Geometry: see drawing. Coordinates: mm, zero at the bounding-box minimum. A direction names the side the tool comes from. Round coordinates to 2 decimals unless told otherwise and drop trailing zeros. Order: outer loops, then holes, each group sorted by start corner. A loop starts at its lowest first (then second) coordinate and runs counter-clockwise, first axis right, second up. Notation, with made-up numbers: (-34, 24) -> (7, 24) arc R21 cw to (7, 36) -> close; hole circle Ø5 at (-32.75, 74). An arc over 180 degrees is marked (long way). Use a Markdown table: item, result.
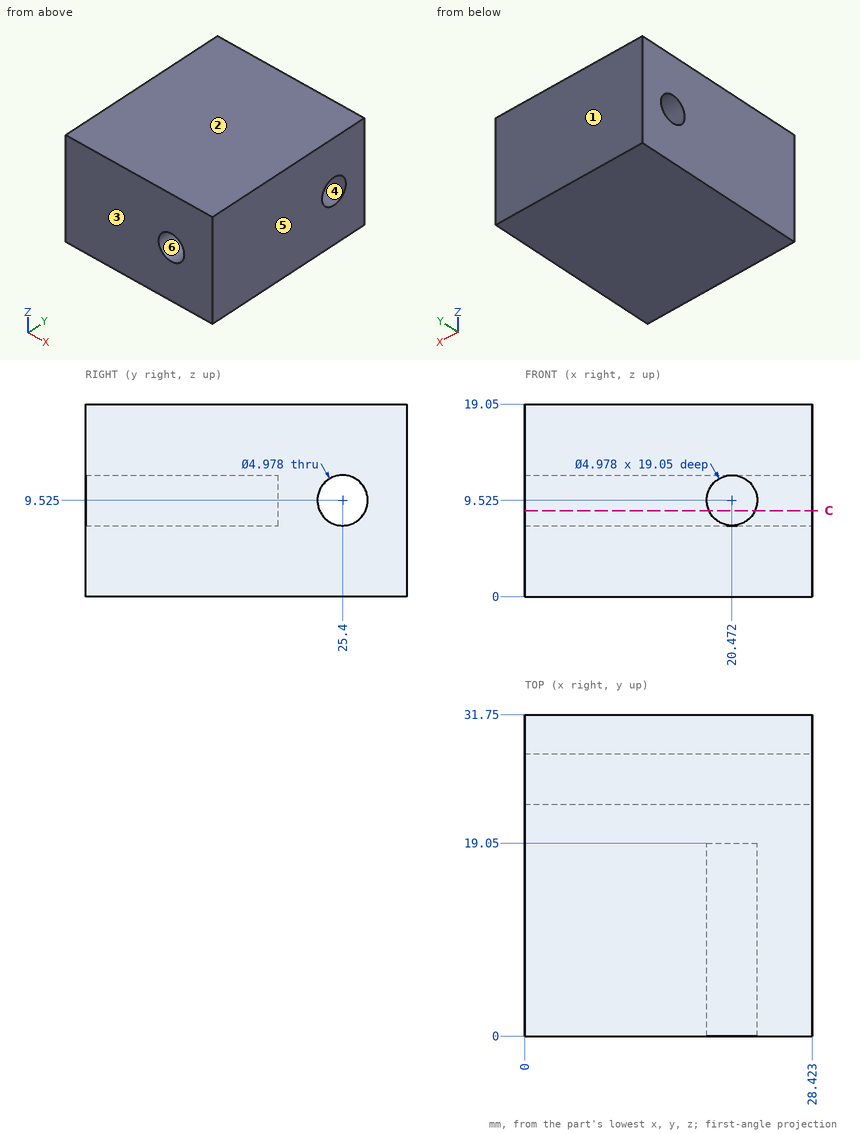
1) Contact query for a flat-ended pin moving along its axis: P1, Ø2.5, axis at x = 19.5, z = 9, coming from the -Y side. Output: stop coordinate, or through.
Answer key:
| item | result |
|---|---|
| P1 | stops at y = 19.05 |
2) Draft query along Y for the marked faces 1, 2, 3 and 4. Return one class per face: released by +Y, released by -Y, zero draft, split by the parting line, or undercut.
Answer key:
| item | result |
|---|---|
| face 1 | released by +Y |
| face 2 | zero draft |
| face 3 | released by -Y |
| face 4 | undercut |
3) Set-up query: the marked faces 5 and 6. Return all of +Z, -Z, +X, -X, +Y, -Y with unobstructed straight access to the full face (end or side cutting, diameter ignored); none if empty.
Answer key:
| item | result |
|---|---|
| face 5 | +Z, -Z, +X, +Y, -Y |
| face 6 | -Y |
4) Ray query, probe 1 along Z at (x, y) = (18.75, 25.5); probe 2 along Y at (x, z) = (12.5, 9); probe 3 along X at (y, z) = (3.5, 9) (1 decimal). Return the intervals inside material, ascending.
Answer key:
| item | result |
|---|---|
| probe 1 | z = 0 to 7.04, 12.01 to 19.05 |
| probe 2 | y = 0 to 22.97, 27.83 to 31.75 |
| probe 3 | x = 0 to 18, 22.9 to 28.4 |
5) Cut plane C-C on z = 8.5. Return loops of the section in (x, y), and give its area (3 significant figures).
Answer key:
| item | result |
|---|---|
| outline | (0, 0) -> (18.2, 0) -> (18.2, 19.05) -> (22.74, 19.05) -> (22.74, 0) -> (28.42, 0) -> (28.42, 23.13) -> (0, 23.13) -> close; (0, 27.67) -> (28.42, 27.67) -> (28.42, 31.75) -> (0, 31.75) -> close |
| area | 687 mm^2 |
